from build123d import *

# Parameters (mm, degrees)
SKETCH_R        = 25
PAD_DEPTH       = 7
PAD001_DEPTH    = 25
CHAMFER_SIZE    = 15
CHAMFER001_SIZE = 10
FILLET_R        = 2
FILLET001_R     = 2
FILLET002_R     = 2
SKETCH002_R     = 1.5
POCKET_DEPTH    = 35.301
FILLET003_R     = 2


with BuildPart() as part:
    # Sketch → Pad (new body)
    with BuildSketch(Plane.XY):
        Circle(SKETCH_R)
    extrude(amount=PAD_DEPTH)

    # Sketch001 → Pad001 (new body)
    with BuildSketch(Plane.XY.offset(7)):
        Polygon((5.3, 21.614464), (10.3, 21.614464), (10.3, 2.5), (24.176399, 2.5), (24.176399, -2.5), (10.3, -2.5), (10.3, -25), (5.3, -25), align=None)
    pad001 = extrude(amount=PAD001_DEPTH)

    # Mirrored: Pad001 across Sketch001 V_Axis
    add(pad001.mirror(Plane(origin=(0, 0, 7), x_dir=(0, 0, 1), z_dir=(1, 0, 0))))

    # Chamfer
    chamfer_edges = [part.edges().sort_by_distance(p)[0] for p in [
        (7.8, 21.614464, 32),
        (-7.8, 21.614464, 32),
    ]]
    chamfer(chamfer_edges, length=CHAMFER_SIZE)

    # Chamfer001
    chamfer001_edges = [part.edges().sort_by_distance(p)[0] for p in [
        (24.176399, 0, 32),
        (-24.176399, 0, 32),
    ]]
    chamfer(chamfer001_edges, length=CHAMFER001_SIZE)

    # Fillet
    fillet_edges = [part.edges().sort_by_distance(p)[0] for p in [
        (10.3, 14.114464, 24.5),
        (10.3, 21.614464, 12),
        (-10.3, 14.114464, 24.5),
        (-10.3, 21.614464, 12),
    ]]
    fillet(fillet_edges, radius=FILLET_R)

    # Fillet001
    fillet001_edges = [part.edges().sort_by_distance(p)[0] for p in [
        (-19.176399, 2.5, 27),
        (-24.176399, 2.5, 14.5),
        (-19.176399, -2.5, 27),
        (-24.176399, -2.5, 14.5),
        (-12.2382, 2.5, 32),
        (-12.2382, -2.5, 32),
    ]]
    fillet(fillet001_edges, radius=FILLET001_R)

    # Fillet002
    fillet002_edges = [part.edges().sort_by_distance(p)[0] for p in [
        (12.2382, 2.5, 32),
        (19.176399, 2.5, 27),
        (24.176399, 2.5, 14.5),
        (24.176399, -2.5, 14.5),
        (19.176399, -2.5, 27),
        (12.2382, -2.5, 32),
    ]]
    fillet(fillet002_edges, radius=FILLET002_R)

    # Sketch002 → Pocket (cut, through all)
    with BuildSketch(Plane.YZ.offset(10.3)):
        with Locations((11.140296, 13.568136)):
            Circle(SKETCH002_R)
        with Locations((-16.31287, 25.611097)):
            Circle(SKETCH002_R)
    extrude(amount=-POCKET_DEPTH, mode=Mode.SUBTRACT)

    # Fillet003
    fillet003_edges = [part.edges().sort_by_distance(p)[0] for p in [
        (-25, 0, 0),
    ]]
    fillet(fillet003_edges, radius=FILLET003_R)


solid = part.part
Model file for the job. Use its own axes, mm. A direction names the side the tool comes from. Round coordinates to 2 decimals unless told otherwise and drop trailing zeros. Loops run counter-clockwise (first coordinate to the right, second up) from the corner with the lowest first, then second, coordinate; pieces in that order, holes last.
1. Band-saw the part on C-C, the plane y = 12. Count the separate pieces of the cut face and the enclosed holes in it, and give its area (3 significant figures).
Check values:
separate pieces: 3
enclosed holes: 0
area: 474 mm2
2. Band-saw the part on A-A, the plane x = 0. List the corners of the cut face in (y, z), and give its area (3 significant figures).
Check values:
outline: (-25, 2) arc R2 ccw to (-23, 0) - (23, 0) arc R2 ccw to (25, 2) - (25, 7) - (-25, 7) - close
area: 348 mm2
3. Mould opens along Y. For faces 1 (the cylindrical face through (-7.765, 12.526, 12.994)), 2 (the flat face through (5.3, -2, 19)), 3 (the cylindrical face through (-12.27, 1.9, 31.43)) say: +Y half, -Y half, draft (parallel to the pull), parting line (faces both ways), or undercut.
Check values:
face 1: undercut
face 2: draft
face 3: +Y half
4. Tool access for faces 4 (the flat face through (16, -2.5, 16)), 5 (the flat face through (8, -24, 7)), 6 (the flat face through (-16, -2.5, 16)), 7 (the cylindrical face through (23.575, 1.93, 14.605)): list every direction of +Z, -Z, +X, -X, +Y, -Y with a clear straight run to the whole face (end or side of a thin tool).
Check values:
face 4: +Z, +X, -Y
face 5: -Z, +X, -Y
face 6: +Z, -X, -Y
face 7: +Z, +X, +Y
5. Band-saw the part on B-B, the plane z = 6. List the corners of the cut face in (x, y), and give its area (3 significant figures).
Check values:
outline: circle Ø50 at (0, 0)
area: 1,960 mm2
6. Wall check: probe 1 along X at (y, z) = (3.5, 17); probe 2 along Y at (x, z) = (-14, 24); probe 3 along Z at (x, y) = (1, 3.5). Give the ranges that are in metal, low to high.
Check values:
probe 1: x = -10.3 to -5.3, 5.3 to 10.3
probe 2: y = -2.5 to 2.5
probe 3: z = 0 to 7
7. Drop flat-ended pins along their axis: P1, Ø9.5, axis at x = 16.5, z = 17, coming from the -Y side; P2, Ø2.5, axis at y = -16.31, z = 25.61, coming from the +X side; P3, Ø1, axis at y = -9.5, z = 28.5, coming from the -X side; P4, Ø0.9, axis at x = -6, z = 12.5, coming from the +Y side. Give the stop position or say it passes through.
Check values:
P1: stops at y = -2.5
P2: passes through
P3: stops at x = -10.3
P4: stops at y = 21.61
